Could you check a few things on this model? Use its own coordinates, in mm. A direction names the side the tool comes from. Coordinates: 2 decimals unless noted, no trailing zeros. Use CSV: the item, a comma, the result in double quotes.
from build123d import *

# Parameters (mm, degrees)
SKETCH1_W           = 47.625
SKETCH1_H           = 47.625
BOSS_EXTRUDE1_DEPTH = 381
BOSS_EXTRUDE1_TAPER = 2.5
SKETCH2_R           = 3.429
CUT_EXTRUDE1_DEPTH  = 381
SKETCH3_W           = 47.625
SKETCH3_H           = 47.625
CUT_EXTRUDE2_DEPTH  = 190.5
SKETCH4_W           = 15.875
SKETCH4_H           = 15.875
CUT_EXTRUDE3_DEPTH  = 6.985
CUT_EXTRUDE3_DRAFT  = -30


with BuildPart() as part:
    # Sketch1 → Boss-Extrude1 (new body)
    with BuildSketch(Plane(origin=(0, 0, 0), x_dir=(1, 0, 0), z_dir=(0, 1, 0))):
        with Locations((23.8125, -23.8125)):
            Rectangle(SKETCH1_W, SKETCH1_H)
    extrude(amount=BOSS_EXTRUDE1_DEPTH, taper=BOSS_EXTRUDE1_TAPER)

    # Sketch2 → Cut-Extrude1 (cut)
    with BuildSketch(Plane.XZ):
        with Locations(Location((23.8125, 23.8125, 0), (0, 0, 270))):
            Circle(SKETCH2_R)
    extrude(amount=-CUT_EXTRUDE1_DEPTH, mode=Mode.SUBTRACT)

    # Sketch3 → Cut-Extrude2 (cut)
    with BuildSketch(Plane.XZ):
        with Locations((23.8125, 23.8125)):
            Rectangle(SKETCH3_W, SKETCH3_H)
    extrude(amount=-CUT_EXTRUDE2_DEPTH, mode=Mode.SUBTRACT)


with BuildPart() as cut_extrude3_tool:
    # Sketch4 → Cut-Extrude3 (with draft: the straight prism first)
    with BuildSketch(Plane.XZ.offset(-190.5)):
        with Locations((23.8125, 23.8125)):
            Rectangle(SKETCH4_W, SKETCH4_H)
    extrude(amount=-CUT_EXTRUDE3_DEPTH)
    # Cut-Extrude3: the draft: its side faces are tilted about the plane it starts from
    cut_extrude3_sides = [cut_extrude3_tool.faces().sort_by_distance(p)[0] for p in [
        (15.875, 193.9925, 23.8125),
        (23.8125, 193.9925, 15.875),
        (31.75, 193.9925, 23.8125),
        (23.8125, 193.9925, 31.75),
    ]]
    draft(cut_extrude3_sides, Plane.XZ.offset(-190.5), CUT_EXTRUDE3_DRAFT)


with BuildPart() as part_1:
    add(part.part)

    # Cut-Extrude3: cut by cut_extrude3_tool
    add(cut_extrude3_tool.part, mode=Mode.SUBTRACT)


solid = part_1.part
(1) Please list where these lines run through material, in increasing order: line 1 (Z direction, x = 26.5, y = 351.5); line 2 (X direction, y = 296.5, z = 21.5); line 3 (X direction, y = 333.5, z = 25.5).
Computed:
line 1,"z = 15.35 to 21.68, 25.94 to 32.28"
line 2,"x = 12.95 to 21.28, 26.34 to 34.68"
line 3,"x = 14.56 to 20.83, 26.8 to 33.06"
(2) Thinking about a two-plate mould opening in Z: for faces 3 (the face through (27.212, 287.958, 24.259)), 4 (the face through (21, 381, 27)), which applies, +Z half, -Z half, draft (parallel to the pull), parting line (faces both ways), or undercut?
Computed:
face 3,"undercut"
face 4,"draft"
(3) Which directions (+Z, -Z, +X, -X, +Y, -Y) give clear straight access to the entire face, cutting with the end or side of a thin tool? Please do faces 1 (the face through (34, 190.5, 24)), 2 (the face through (30.21, 193.17, 23.7)).
Computed:
face 1,"+Z, -Z, +X, -X, -Y"
face 2,"-Y"
(4) Will these pins go through, and if not, where does the flat tip stop? pin 1 (1 mm diameter, centred on y = 219, z = 22, fed in from +X); pin 2 (8 mm diameter, centred on x = 21, y = 294.5, fed in from -Z); pin 3 (1.5 mm diameter, centred on y = 217.5, z = 23, fed in from +X).
Computed:
pin 1,"stops at x = 38.09"
pin 2,"stops at z = 12.68"
pin 3,"stops at x = 38.16"
